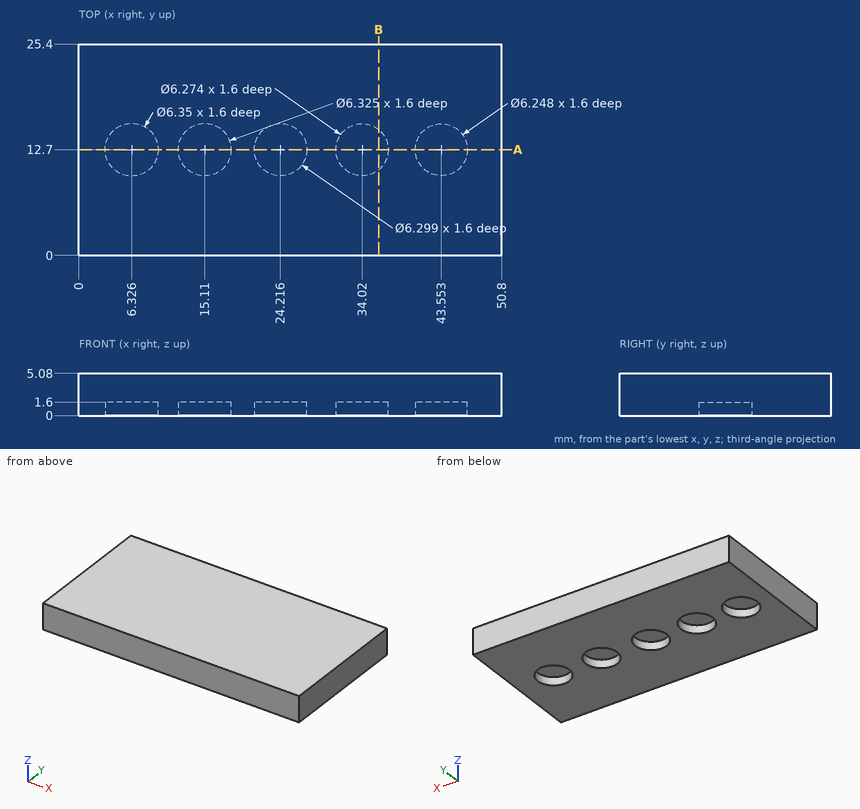
Verification items for this drawing (mm, ordinates from the low corner). Give positions to 0.01 mm unless a question says otherwise; leave off trailing zeros. Loops run counter-clockwise (first coordinate to the right, second up) from the corner with the lowest first, then second, coordinate; pieces in that order, holes last. Notation, with made-up numbers: M 29,27 L 61,27 A12 ccw 61,38 Z; hole C 15.5,39.5 d4. An arc over 180 degrees is marked long. Answer in a Markdown table with one row per item.
1) Thickness scan on line 1 (X direction, y = 12.7, z = 1.2); line 2 (Y direction, x = 17.5, z = 1.55); line 3 (Z direction, x = 23, y = 13.75). Record the ranges inside material, lowest first.
Solutions:
| item | result |
|---|---|
| line 1 | x = 0 to 3.15, 9.5 to 11.95, 18.27 to 21.07, 27.37 to 30.88, 37.16 to 40.43, 46.68 to 50.8 |
| line 2 | y = 0 to 10.63, 14.77 to 25.4 |
| line 3 | z = 1.6 to 5.08 |
2) Cross-section at A-A (y = 12.7). Enter the section's corners in (x, z).
Solutions:
| item | result |
|---|---|
| outline | M 0,0 L 3.15,0 L 3.15,1.6 L 9.5,1.6 L 9.5,0 L 11.95,0 L 11.95,1.6 L 18.27,1.6 L 18.27,0 L 21.07,0 L 21.07,1.6 L 27.37,1.6 L 27.37,0 L 30.88,0 L 30.88,1.6 L 37.16,1.6 L 37.16,0 L 40.43,0 L 40.43,1.6 L 46.68,1.6 L 46.68,0 L 50.8,0 L 50.8,5.08 L 0,5.08 Z |
3) Depth check by flat-ended pin: pin 1 (1.9 mm diameter, centred on x = 44, y = 12, fed in from -Z). Enter the tip coordinate at first touch or a pass-through.
Solutions:
| item | result |
|---|---|
| pin 1 | stops at z = 1.6 |
4) Cross-section at B-B (x = 36). Enter the section's corners in (y, z), plus the area to 3 significant figures.
Solutions:
| item | result |
|---|---|
| outline | M 0,0 L 10.27,0 L 10.27,1.6 L 15.13,1.6 L 15.13,0 L 25.4,0 L 25.4,5.08 L 0,5.08 Z |
| area | 121 mm^2 |
